from build123d import *

# Parameters (mm, degrees)
EXTRUDE_1_DEPTH = 5
FILLET_1_R      = 10


with BuildPart() as part:
    # Эскиз1 → Бобышка-Вытянуть1 (new body)
    with BuildSketch(Plane(origin=(0, 0, 0), x_dir=(1, 0, 0), z_dir=(0, 1, 0))):
        with BuildLine():
            Line((-12.727922061, 12.727922061), (-45.961940777, 45.961940777))
            ThreePointArc((-45.961940777, 45.961940777), (24.874423104, -60.052169613), (0, 65))
            Line((0, 65), (0, 18))
            ThreePointArc((0, 18), (6.888301783, -16.629831585), (-12.727922061, 12.727922061))
        make_face()
    extrude(amount=EXTRUDE_1_DEPTH)

    # Скругление1
    fillet_1_edges = [part.edges().sort_by_distance(p)[0] for p in [
        (-45.961940777, 2.5, -45.961940777),
    ]]
    fillet(fillet_1_edges, radius=FILLET_1_R)


solid = part.part
Source: CAD feature listing. Evaluate the final solid. Frame: model axes, mm. A direction names the side the tool comes from. Round coordinates to 2 decimals unless told otherwise and drop trailing zeros. Loops run counter-clockwise (first coordinate to the right, second up) from the corner with the lowest first, then second, coordinate; pieces in that order, holes last. Notation, with made-up numbers: (77.25, 51) -> (123.25, 51) arc R11 cw to (123.25, 62) -> close; hole circle Ø4 at (31, -37). An arc over 180 degrees is marked (long way). Answer as a JSON object with one key per item and string values. Group by question number.
Q1. Section query C-C (z = -22.5). Output: boundary loops of the cut face in (x, y), plus the area to 3 significant figures.
Q2. Section query B-B (y = 2.7). Output: boundary loops of the cut face in (x, z).
Q3. Contact query for flat-ended pins moving along their axis: P1, Ø8, axis at x = -26, z = -12.5, coming from the -Y side; P2, Ø3, axis at x = -13.5, y = 0.5, coming from the -Z side; P3, Ø2.5, axis at y = 3, z = -32, coming from the -X side; P4, Ø2, axis at y = 3.5, z = -40, coming from the -X side. Output: stop coordinate, or through.
Q4. Section query A-A (z = 0). Output: boundary loops of the cut face in (x, y), plus the area to 3 significant figures.
Q5. Mould query, pull axis X, two halves, no side actions, for faces 1 (the cylindrical face through (28.092, 2.465, 58.616)), 2 (the cylindrical face through (-46.1, 2.54, -41.14)), 3 (the flat face through (14, 5, 14)). Classes: pulls with the +X half, pulls with the -X half, needs draft (parallel to the pull), parting line crosses it, or undercut.
Q6. Section query D-D (z = 25). Output: boundary loops of the cut face in (x, y), plus the area to 3 significant figures.
Q7. Ray query, line 1 (X direction, y = 1.1, z = 0); line 2 (Z direction, x = -15, y = 2); line 3 (Z direction, x = 12, y = 1.1). Return the intervals inside material, ascending. Write a range as from..to.
Q8. Access query for faces 4 (the cylindrical face through (7.523, 2.465, 16.352)), 5 (the flat face through (-25, 2, -25)). Directions: +Z, -Z, +X, -X, +Y, -Y. A direction counts if a zero-diameter tool reaches every point of the face in a straight line with its end or side. Return the directions, or none.
Completed:
{
 "1": {"outline": "(-60.98, 0) -> (-22.5, 0) -> (-22.5, 5) -> (-60.98, 5) -> close; (0, 0) -> (60.98, 0) -> (60.98, 5) -> (0, 5) -> close", "area": "497 mm²"},
 "2": {"outline": "(-53.55, -36.84) arc R10 ccw to (-38.24, -38.24) -> (-12.73, -12.73) arc R18 cw (long way) to (0, -18) -> (0, -65) arc R65 ccw (long way) to start"},
 "3": {"P1": "y = 0", "P2": "z = -15", "P3": "x = -57.27", "P4": "x = -51.54"},
 "4": {"outline": "(-65, 0) -> (-18, 0) -> (-18, 5) -> (-65, 5) -> close; (18, 0) -> (65, 0) -> (65, 5) -> (18, 5) -> close", "area": "470 mm²"},
 "5": {"face 1": "parting line crosses it", "face 2": "undercut", "face 3": "needs draft"},
 "6": {"outline": "(-60, 0) -> (60, 0) -> (60, 5) -> (-60, 5) -> close", "area": "600 mm²"},
 "7": {"line 1": "-65..-18, 18..65", "line 2": "-15..-9.95, 9.95..63.25", "line 3": "-63.88..-13.42, 13.42..63.88"},
 "8": {"face 4": "+Y, -Y", "face 5": "-Z, +Y, -Y"}
}
